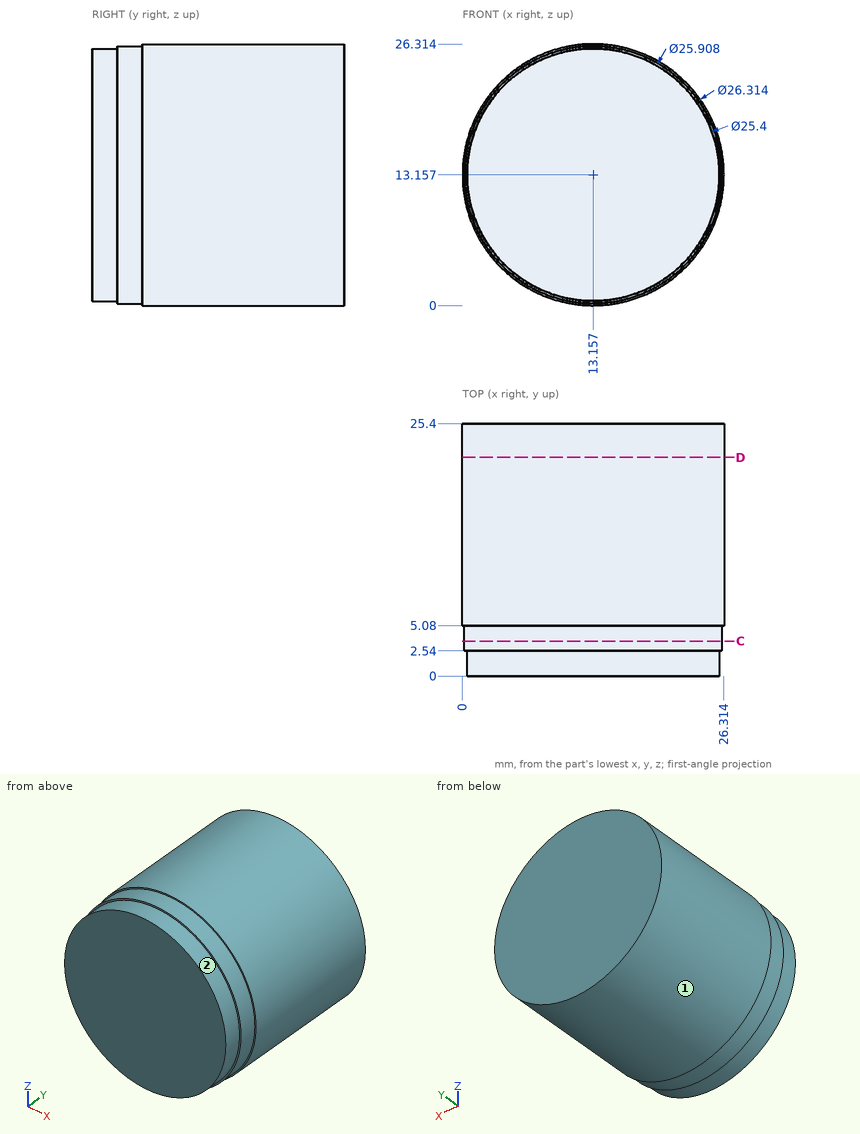
Geometry check sheet. Reference: drawing and pictorial views, mm from the part's lowest x, y, z. A direction names the side the tool comes from. Round coordinates to 2 decimals unless told otherwise and drop trailing zeros. Order: outer loops, then holes, each group sorted by start corner. A loop starts at its lowest first (then second) coordinate and runs counter-clockwise, first axis right, second up. Notation, with made-up numbers: (-9.75, 51.25) - (11.25, 51.25) arc R22 ccw to (11.25, 87.25) - close; hole circle Ø7 at (83.5, -32.75). An arc over 180 degrees is marked (long way). Write item = value, one per line.
Q1. Thickness scan on line 1 along X through (y, z) = (2, 8.25) (1 decimal); line 2 along X through (y, z) = (16.75, 21.5) (1 decimal). Record the ranges inside material, lowest first.
Computed:
line_1 = 1.4 to 24.9
line_2 = 3 to 23.3
Q2. Section check C-C (y = 3.5). Record the boundary of the cut face in (x, z), and give its area (3 significant figures).
Computed:
outline = circle Ø25.91 at (13.16, 13.16)
area = 527 mm^2
Q3. Section check D-D (y = 22). Record the boundary of the cut face in (x, z) (1 decimal).
Computed:
outline = circle Ø26.3 at (13.2, 13.2)
Q4. Tool access check on the marked faces 1 and 2. Record the directions out of +Z, -Z, +X, -X, +Y, -Y that give a thin tool (end or side, any length) a straight path to the whole face; none if there is none.
Computed:
face_1 = +Y, -Y
face_2 = -Y
Q5. Go/stop test with flat-tipped pins: pin 1 (4 mm diameter, centred on x = 9, y = 11.5, fed in from +Z); pin 2 (4 mm diameter, centred on y = 13, z = 6.5, fed in from +X); pin 3 (1 mm diameter, centred on x = 9, y = 14.5, fed in from +Z). Record where each tip stops, or that it passes through.
Computed:
pin_1 = 26.14
pin_2 = 25.46
pin_3 = 25.8
